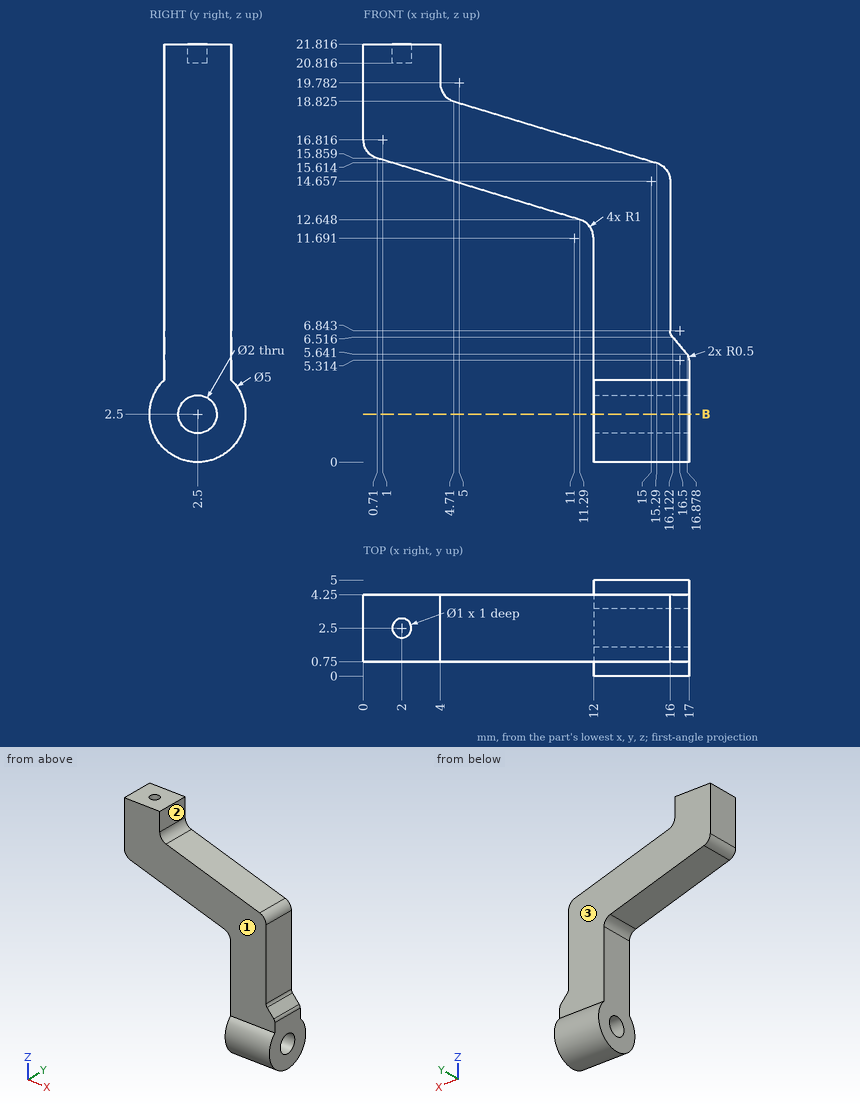
Verification items for this drawing (mm, ordinates from the low corner). A direction names the side the tool comes from. Give positions to 0.01 mm unless a question says otherwise; leave off trailing zeros. Write each loop counter-clockwise with the first axis right and the second up, starting at its lowest first coordinate (ties: lowest second). Pieces come first, ordered by that corner, then holes. Notation, with made-up numbers: (40, 89) -> (60, 89) arc R15 cw to (60, 99) -> close; hole circle Ø3 at (16.25, -22.5). An arc over 180 degrees is marked (long way). Use one line per item in the form item = value.
Item 1: Access from +Z, -Z, +X, -X, +Y, -Y to the whole of each face (thin tool, end or side, straight path). Record for the marked faces 1, 2 and 3.
Results list:
face_1 = +Z, +X, -X, -Y
face_2 = +Z, +X, +Y, -Y
face_3 = +Z, +X, -X, +Y
Item 2: Depth check by flat-ended pin: pin 1 Ø1.6 at (y, z) = (1.5, 20.5) entering from +X; pin 2 Ø1 at (y, z) = (3, 11) entering from +X; pin 3 Ø2 at (x, z) = (7, 16.5) entering from +Y. Enter the tip coordinate at first touch or a pass-through.
Results list:
pin_1 = 4
pin_2 = 16
pin_3 = 4.25
Item 3: Sectioned sample at B-B on z = 2.5. Enter the section's corners in (x, y), plus the area to 3 significant figures.
Results list:
outline = (12, 0) -> (17, 0) -> (17, 1.5) -> (12, 1.5) -> close; (12, 3.5) -> (17, 3.5) -> (17, 5) -> (12, 5) -> close
area = 15.0 mm2
Item 4: Scan lines: line 1 (Y direction, x = 15.3, z = 2.5); line 2 (X direction, y = 4.1, z = 7); line 3 (Y direction, x = 13.75, z = 6). Record each from-to range of solid material in increasing order.
Results list:
line_1 = 0 to 1.5, 3.5 to 5
line_2 = 12 to 16
line_3 = 0.75 to 4.25
